from build123d import *

# Parameters (mm, degrees)
SKETCH1_R          = 300
PLATE_DEPTH        = 15
SKETCH2_R          = 87.5
BEARING_HOLE_DEPTH = 425.529150943
SKETCH4_R          = 280
SKETCH4_R_2        = 275
CUT_EXTRUDE3_DEPTH = 10


with BuildPart() as part:
    # Sketch1 → plate (new body)
    with BuildSketch(Plane(origin=(0, 0, 0), x_dir=(1, 0, 0), z_dir=(0, 1, 0))):
        with Locations(Location((0, 0, 0), (0, 0, 270))):
            Circle(SKETCH1_R)
    extrude(amount=PLATE_DEPTH)

    # Sketch2 → bearing-hole (cut, through all)
    with BuildSketch(Plane(origin=(0, 15, 0), x_dir=(1, 0, 0), z_dir=(0, 1, 0))):
        with Locations(Location((0, 0, 0), (0, 0, 270))):
            Circle(SKETCH2_R)
    extrude(amount=-BEARING_HOLE_DEPTH, mode=Mode.SUBTRACT)

    # Sketch4 → Cut-Extrude3 (cut)
    with BuildSketch(Plane(origin=(0, 15, 0), x_dir=(1, 0, 0), z_dir=(0, 1, 0))):
        with Locations(Location((0, 0, 0), (0, 0, 270))):
            Circle(SKETCH4_R)
        with Locations(Location((0, 0, 0), (0, 0, 270))):
            Circle(SKETCH4_R_2, mode=Mode.SUBTRACT)
    extrude(amount=-CUT_EXTRUDE3_DEPTH, mode=Mode.SUBTRACT)


solid = part.part
Work out the finished part from the listing and answer in its coordinate system (mm). A direction names the side the tool comes from. Give positions to 0.01 mm unless a question says otherwise; leave off trailing zeros. Order: outer loops, then holes, each group sorted by start corner. A loop starts at its lowest first (then second) coordinate and runs counter-clockwise, first axis right, second up. Notation, with made-up numbers: (4, 42) -> (36, 42) arc R25 ccw to (36, 74) -> close; hole circle Ø9 at (-27, 88.5). An arc over 180 degrees is marked (long way). One line per item, written item: value.
Item 1: A tool of negligible diameter and unlimited length cuts with its end or side. For faces 4 (the flat face through (-62, 0, 62)), 5 (the cylindrical face through (-170.376, 10.07, -222.198)), from which of +Z, -Z, +X, -X, +Y, -Y can it reach the whole face along a straight path? Write none if from no direction.
Answer sheet:
face 4: +Z, -Z, +X, -X, -Y
face 5: +Y
Item 2: Find section B-B, the plane z = 0. Give the vertices of the cut face in (x, y).
Answer sheet:
outline: (-300, 0) -> (-87.5, 0) -> (-87.5, 15) -> (-275, 15) -> (-275, 5) -> (-280, 5) -> (-280, 15) -> (-300, 15) -> close; (87.5, 0) -> (300, 0) -> (300, 15) -> (280, 15) -> (280, 5) -> (275, 5) -> (275, 15) -> (87.5, 15) -> close
Item 3: Find section A-A, the plane x = 0. Give the vertices of the cut face in (y, z).
Answer sheet:
outline: (0, -300) -> (15, -300) -> (15, -280) -> (5, -280) -> (5, -275) -> (15, -275) -> (15, -87.5) -> (0, -87.5) -> close; (0, 87.5) -> (15, 87.5) -> (15, 275) -> (5, 275) -> (5, 280) -> (15, 280) -> (15, 300) -> (0, 300) -> close
Item 4: Straight lines are drawn through the part: probe 1 along X at (y, z) = (5.5, 0); probe 2 along X at (y, z) = (3, 0); probe 3 along X at (y, z) = (12.5, -249). For each, find the intervals that lie inside material, in ascending order.
Answer sheet:
probe 1: -300 to -280, -275 to -87.5, 87.5 to 275, 280 to 300
probe 2: -300 to -87.5, 87.5 to 300
probe 3: -167.33 to -128.06, -116.72 to 116.72, 128.06 to 167.33
Item 5: Find section C-C, the plane x = -115.5. Give the vertices of the cut face in (y, z), plus the area to 3 significant figures.
Answer sheet:
outline: (0, -276.87) -> (15, -276.87) -> (15, -255.07) -> (5, -255.07) -> (5, -249.57) -> (15, -249.57) -> (15, 249.57) -> (5, 249.57) -> (5, 255.07) -> (15, 255.07) -> (15, 276.87) -> (0, 276.87) -> close
area: 8,200 mm²
Item 6: Flat-ended cylindrical pins translate along their axes: P1, Ø2, axis at y = 10.5, z = -230.5, coming from the -X side; P2, Ø3, axis at y = 2.5, z = -109.5, coming from the -X side; P3, Ø6, axis at x = 231, y = 4, coming from the +Z side. Find the tip coordinate at first contact, or state that the pin passes through.
Answer sheet:
P1: x = -193.21
P2: x = -279.89
P3: z = 194.98
Item 7: Determine the mould class of faces 1 (the flat face through (-206, 5, 185)), 2 (the cylindrical face through (-182.545, 7.395, -238.07)), 3 (the flat face through (135, 15, -246)) for opening direction X: released by +X, released by -X, zero draft, split by the parting line, or undercut.
Answer sheet:
face 1: undercut
face 2: split by the parting line
face 3: zero draft
Item 8: Find section D-D, the plane z = 215. Give the vertices of the cut face in (x, y), plus the area to 3 significant figures.
Answer sheet:
outline: (-209.22, 0) -> (209.22, 0) -> (209.22, 15) -> (179.37, 15) -> (179.37, 5) -> (171.46, 5) -> (171.46, 15) -> (-171.46, 15) -> (-171.46, 5) -> (-179.37, 5) -> (-179.37, 15) -> (-209.22, 15) -> close
area: 6,120 mm²
